Geometry: final body of the model. Coordinates: model frame, mm. Round coordinates to 2 decimals unless told otherwise and drop trailing zeros. Loops run counter-clockwise (first coordinate to the right, second up) from the corner with the lowest first, then second, coordinate; pieces in that order, holes last. Notation, with made-up numbers: (39.25, 59) - (61.25, 59) arc R14 cw to (61.25, 76) - close; hole circle Ø5 at (79.5, 16.25). An arc over 180 degrees is marked (long way). Return JSON: item names as keys, results as strings. Group by question number.
1. Section D-D on x = 166.2. Return loops of the section in (y, z), and give its area (3 significant figures).
2. First-contact query: pin 1 Ø4.5 at (x, y) = (51.9, 105.4) entering from +Z. Flat tip, straight axial feed; report the tip coordinate or a pass-through.
3. Section B-B on x = 51.9. Return loops of the section in (y, z).
4. Section A-A on y = 34. Return loops of the section in (x, z), and give its area (3 significant figures).
5. Material intervals for probe 1 along Y at (x, z) = (51.9, 2); probe 2 along X at (y, z) = (79, 2); probe 3 along X at (y, z) = (14.5, 1.5), sorted ascending.
6. Section C-C on y = 94. Return loops of the section in (x, z).
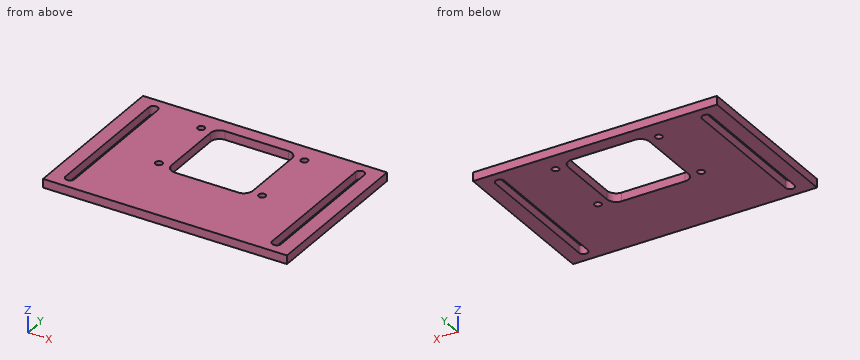
from build123d import *

# Parameters (mm, degrees)
F0_W     = 180
F0_H     = 120
F1_DEPTH = 6.35
F3_DEPTH = 6.351
F4_W     = 30
F4_H     = 20
F5_DEPTH = 6.351
F7_D     = 5.1054


with BuildPart() as f1:
    # F0 (on Top) → F1 (new body)
    with BuildSketch(Plane.XY):
        with Locations((90, 60)):
            Rectangle(F0_W, F0_H)
    extrude(amount=F1_DEPTH)

    # F2 (on face) → F3 (cut, through all)
    with BuildSketch(Plane.XY.offset(6.35)):
        with BuildLine():
            Line((10.498, 110), (10.498, 60))
            Line((10.498, 60), (13.8, 60))
            Line((13.8, 60), (17.102, 60))
            Line((17.102, 60), (17.102, 110))
            ThreePointArc((17.102, 110), (13.8, 113.302), (10.498, 110))
        make_face()
        with BuildLine():
            Line((162.898, 110), (162.898, 60))
            Line((162.898, 60), (166.2, 60))
            Line((166.2, 60), (169.502, 60))
            Line((169.502, 60), (169.502, 110))
            ThreePointArc((169.502, 110), (166.2, 113.302), (162.898, 110))
        make_face()
        with BuildLine():
            Line((166.2, 60), (162.898, 60))
            Line((162.898, 60), (162.898, 10))
            ThreePointArc((162.898, 10), (166.2, 6.698), (169.502, 10))
            Line((169.502, 10), (169.502, 60))
            Line((169.502, 60), (166.2, 60))
        make_face()
        with BuildLine():
            Line((13.8, 60), (10.498, 60))
            Line((10.498, 60), (10.498, 10))
            ThreePointArc((10.498, 10), (13.8, 6.698), (17.102, 10))
            Line((17.102, 10), (17.102, 60))
            Line((17.102, 60), (13.8, 60))
        make_face()
    extrude(amount=-F3_DEPTH, mode=Mode.SUBTRACT)

    # F4 (on face) → F5 (cut, through all)
    with BuildSketch(Plane.XY.offset(6.35)):
        with BuildLine():
            Line((113.396, 110), (90, 110))
            Line((90, 110), (90, 80))
            Line((90, 80), (120, 80))
            Line((120, 80), (120, 103.396))
            ThreePointArc((120, 103.396), (118.065733183, 108.065733183), (113.396, 110))
        make_face()
        with BuildLine():
            Line((90, 80), (90, 110))
            Line((90, 110), (66.604, 110))
            ThreePointArc((66.604, 110), (61.934266817, 108.065733183), (60, 103.396))
            Line((60, 103.396), (60, 80))
            Line((60, 80), (90, 80))
        make_face()
        with Locations((105, 70)):
            Rectangle(F4_W, F4_H)
        with Locations((75, 70)):
            Rectangle(F4_W, F4_H)
        with BuildLine():
            Line((120, 60), (90, 60))
            Line((90, 60), (90, 50))
            Line((90, 50), (113.396, 50))
            ThreePointArc((113.396, 50), (118.065733183, 51.934266817), (120, 56.604))
            Line((120, 56.604), (120, 60))
        make_face()
        with BuildLine():
            Line((90, 50), (90, 60))
            Line((90, 60), (60, 60))
            Line((60, 60), (60, 56.604))
            ThreePointArc((60, 56.604), (61.934266817, 51.934266817), (66.604, 50))
            Line((66.604, 50), (90, 50))
        make_face()
    extrude(amount=-F5_DEPTH, mode=Mode.SUBTRACT)

    # F7 (through all)
    with Locations(Plane.XY.offset(6.35)):
        with Locations((51.9, 105.4), (128.1, 105.4), (128.1, 54.6), (51.9, 54.6)):
            Hole(F7_D / 2)


solid = f1.part
Taken from the geometry:
{
 "1": {"outline": "(0, 0) - (6.7, 0) - (6.7, 6.35) - (0, 6.35) - close; (113.3, 0) - (120, 0) - (120, 6.35) - (113.3, 6.35) - close", "area": "85.1 mm2"},
 "2": {"pin 1": "through"},
 "3": {"outline": "(0, 0) - (52.05, 0) - (52.05, 6.35) - (0, 6.35) - close; (57.15, 0) - (102.85, 0) - (102.85, 6.35) - (57.15, 6.35) - close; (107.95, 0) - (120, 0) - (120, 6.35) - (107.95, 6.35) - close"},
 "4": {"outline": "(0, 0) - (10.5, 0) - (10.5, 6.35) - (0, 6.35) - close; (17.1, 0) - (162.9, 0) - (162.9, 6.35) - (17.1, 6.35) - close; (169.5, 0) - (180, 0) - (180, 6.35) - (169.5, 6.35) - close", "area": "1,060 mm2"},
 "5": {"probe 1": "0 to 52.05, 57.15 to 102.85, 107.95 to 120", "probe 2": "0 to 10.5, 17.1 to 60, 120 to 162.9, 169.5 to 180", "probe 3": "0 to 10.5, 17.1 to 162.9, 169.5 to 180"},
 "6": {"outline": "(0, 0) - (10.5, 0) - (10.5, 6.35) - (0, 6.35) - close; (17.1, 0) - (60, 0) - (60, 6.35) - (17.1, 6.35) - close; (120, 0) - (162.9, 0) - (162.9, 6.35) - (120, 6.35) - close; (169.5, 0) - (180, 0) - (180, 6.35) - (169.5, 6.35) - close"}
}
